Autodesk Fusion 360 part; units mm, degrees
sketch "Sketch1" plane through (0, 0, 0) normal (0, 0, 1) x (1, 0, 0)
  circle A0 centre (0, 0) radius 11
  circle A1 centre (0, 0) radius 22.5
  circle A2 centre (0, 0) radius 38
  dimension "d1" = 45
  dimension "d2" = 22
  dimension "d3" = 76
extrude "Extrude1" add sketch "Sketch1" along normal blind 20 contours A1
sketch "Sketch2" plane through (0, 0, 0) normal (0, 0, 1) x (1, 0, 0)
  circle A0 centre (0.2654, -30.1553) radius 2.5
  dimension "d8" = 5
extrude "Extrude4" add sketch "Sketch1" along normal blind 2 contours A1 | A2
extrude "Extrude5" cut sketch "Sketch2" along normal blind 6.312
pattern_circular "C-Pattern2" count 3 over 360 about axis through (0, 0, 2) along (0, 0, 1) of "Extrude5"
extrude "돌출6" add 1 faces at (-20.8034, 21.3677, 2) along direction (0, 0, 1) blind 20
extrude "돌출7" cut 1 faces at (-20.8034, 21.3677, 22) along direction (0, 0, -1) blind 3
extrude "돌출8" add 1 faces at (-20.8034, 21.3677, 19) along direction (0, 0, 1) blind 1
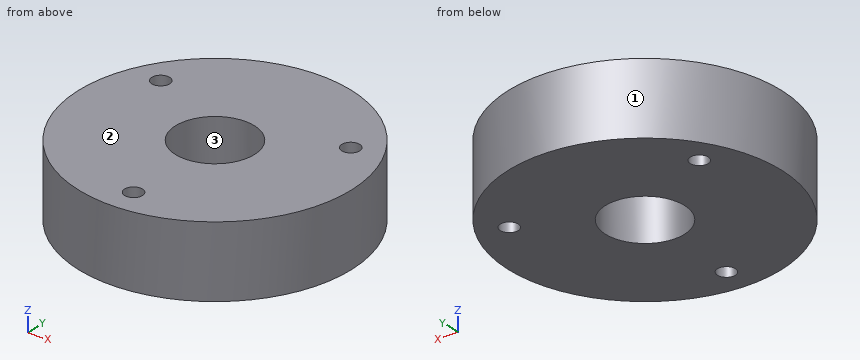
CAD build for the part. Positions are in the model's coordinates, mm. Face numbers are marked on the shaded views. Round coordinates to 2 decimals unless told otherwise and drop trailing zeros. Write each loop counter-clockwise with the first axis right and the second up, starting at its lowest first coordinate (ties: lowest second). Pieces come first, ordered by that corner, then holes. Notation, with made-up numbers: (-20, 51) -> (35, 51) arc R32 ccw to (35, 85) -> close; hole circle Ø4 at (24.25, 1.5). An arc over 180 degrees is marked (long way). Answer in a Markdown table with one row per item. Add a question column.
Item 1: Drop flat-ended pins along their axis: pin 1 Ø6 at (y, z) = (-7.5, 6.5) entering from +X; pin 2 Ø1 at (y, z) = (14.5, 15) entering from -X; pin 3 Ø3 at (x, y) = (0.27, -30.16) entering from +Z; pin 4 Ø3 at (y, z) = (-13, 8.5) entering from +X. Give the stop position or say it passes through.
Item 2: Saw through at C-C, the plane x = 0. Write the cut outline in (y, z), then the cut area to 3 significant figures.
Item 3: Saw through at B-B, the plane x = 8. Write the cut outline in (y, z), then the cut area to 3 significant figures.
Item 4: Saw through at A-A, the plane y = 0. Write the cut outline in (x, z), then the cut area to 3 significant figures.
Item 5: Mould opens along X. For the marked faces 1, 2 and 3 say: pulls with the +X half, pulls with the -X half, needs draft (parallel to the pull), parting line crosses it, or undercut.
Item 6: Drill centre lines: line 1 (Y direction, x = 0, z = 14.5); line 2 (X direction, y = 14, z = 2.5); line 3 (Y direction, x = 1, z = 3.75). Where is each one in solid material? Low to high. Write a range as from..to.
Item 7: Saw through at D-D, the plane z = 7.25. Write the cut outline in (x, y), then the cut area to 3 significant figures.
Findings below:
| question | item | result |
|---|---|---|
| 1 | pin 1 | stops at x = 37.73 |
| 1 | pin 2 | stops at x = -35.33 |
| 1 | pin 3 | passes through |
| 1 | pin 4 | stops at x = 36.22 |
| 2 | outline | (-38, 0) -> (-32.64, 0) -> (-32.64, 20) -> (-38, 20) -> close; (-27.67, 0) -> (-11, 0) -> (-11, 20) -> (-27.67, 20) -> close; (11, 0) -> (38, 0) -> (38, 20) -> (11, 20) -> close |
| 2 | area | 981 mm^2 |
| 3 | outline | (-37.15, 0) -> (-7.55, 0) -> (-7.55, 20) -> (-37.15, 20) -> close; (7.55, 0) -> (37.15, 0) -> (37.15, 20) -> (7.55, 20) -> close |
| 3 | area | 1,180 mm^2 |
| 4 | outline | (-38, 0) -> (-11, 0) -> (-11, 20) -> (-38, 20) -> close; (11, 0) -> (38, 0) -> (38, 20) -> (11, 20) -> close |
| 4 | area | 1,080 mm^2 |
| 5 | face 1 | parting line crosses it |
| 5 | face 2 | needs draft |
| 5 | face 3 | undercut |
| 6 | line 1 | y = -38..-32.64, -27.67..-11, 11..38 |
| 6 | line 2 | x = -35.33..-28.6, -23.9..23.85, 28.11..35.33 |
| 6 | line 3 | y = -37.99..-32.54, -27.77..-10.95, 10.95..37.99 |
| 7 | outline | circle Ø76 at (0, 0); hole circle Ø5 at (-26.25, 14.85); hole circle Ø22 at (0, 0); hole circle Ø5 at (0.27, -30.16); hole circle Ø5 at (25.98, 15.31) |
| 7 | area | 4,100 mm^2 |
